from build123d import *

# Parameters (mm, degrees)
SKETCH1_R           = 15
BOSS_EXTRUDE1_DEPTH = 5
SKETCH3_R           = 18.5
SKETCH3_R_2         = 15
BOSS_EXTRUDE3_DEPTH = 1
SKETCH2_R           = 7.5
BOSS_EXTRUDE2_DEPTH = 0.5
BOSS_EXTRUDE5_DEPTH = 5.5
BOSS_EXTRUDE6_START = 0.5
BOSS_EXTRUDE6_DEPTH = 0.5


with BuildPart() as part:
    # Sketch1 → Boss-Extrude1 (new, symmetric)
    with BuildSketch(Plane.XY):
        with Locations((-2.17, 0)):
            Circle(SKETCH1_R)
        Polygon((-2, 3.464101615), (-4, 0), (-2, -3.464101615), (2, -3.464101615), (4, 0), (2, 3.464101615), align=None, mode=Mode.SUBTRACT)
    extrude(amount=BOSS_EXTRUDE1_DEPTH, both=True)

    # Sketch3 → Boss-Extrude3 (add)
    # profile 1 of 2: a face of its own
    with BuildSketch(Plane(origin=(0, 0, -5), x_dir=(-1, 0, 0), z_dir=(0, 0, -1))):
        with Locations((2.17, 0)):
            Circle(SKETCH3_R)
        with Locations(Location((2.17, 0, 0), (0, 0, 180))):
            Circle(SKETCH3_R_2, mode=Mode.SUBTRACT)
    # profile 2 of 2: a face of its own
    with BuildSketch(Plane(origin=(0, 0, -5), x_dir=(-1, 0, 0), z_dir=(0, 0, -1))):
        with Locations(Location((2.17, 0, 0), (0, 0, 180))):
            Circle(SKETCH3_R_2)
        Polygon((-4, 0), (-2, 3.464101615), (2, 3.464101615), (4, 0), (2, -3.464101615), (-2, -3.464101615), align=None, mode=Mode.SUBTRACT)
    extrude(amount=BOSS_EXTRUDE3_DEPTH)

    # Sketch2 → Boss-Extrude2 (add)
    with BuildSketch(Plane(origin=(0, 0, -6), x_dir=(-1, 0, 0), z_dir=(0, 0, -1))):
        Circle(SKETCH2_R)
        Polygon((2, -3.464101615), (-2, -3.464101615), (-4, 0), (-2, 3.464101615), (2, 3.464101615), (4, 0), align=None, mode=Mode.SUBTRACT)
    extrude(amount=BOSS_EXTRUDE2_DEPTH)

    # Sketch4 → Boss-Extrude5 (add)
    with BuildSketch(Plane.XY.offset(5)):
        Polygon((4, 6.92820323), (-4, 6.92820323), (-8, 0), (-4, -6.92820323), (4, -6.92820323), (8, 0), align=None)
    extrude(amount=BOSS_EXTRUDE5_DEPTH)

    # Sketch5 → Boss-Extrude6 (add)
    with BuildSketch(Plane.XY.offset(5).offset(BOSS_EXTRUDE6_START)):
        with BuildLine():
            ThreePointArc((-13.508064516, -9.820809184), (-7.396562926, -14.059980085), (0, -14.842206709))
            Line((0, -14.842206709), (0, -6.92820323))
            Line((0, -6.92820323), (-4, -6.92820323))
            Line((-4, -6.92820323), (-8, 0))
            Line((-8, 0), (-4, 6.92820323))
            Line((-4, 6.92820323), (0, 6.92820323))
            Line((0, 6.92820323), (0, 14.842206709))
            ThreePointArc((0, 14.842206709), (-7.396562926, 14.059980085), (-13.508064516, 9.820809184))
            ThreePointArc((-13.508064516, 9.820809184), (-16.33, 0), (-13.508064516, -9.820809184))
        make_face()
    extrude(amount=-BOSS_EXTRUDE6_DEPTH)


solid = part.part
Input: part model. Units: mm. Frame: model coordinates. A direction names the side the tool comes from. Coordinates: 2 decimals unless noted, no trailing zeros. Loops run counter-clockwise (first coordinate to the right, second up) from the corner with the lowest first, then second, coordinate; pieces in that order, holes last. Notation, with made-up numbers: (56, 35) -> (91, 35) arc R14 ccw to (91, 45) -> close; hole circle Ø9 at (-8.5, 8). An arc over 180 degrees is marked (long way). Write item = value, one per line. Start each with the question number.
Item 1: Reachability of faces 5 (the face through (-8.3, 0.2, 5.5)), 6 (the face through (-6.028, -3.416, 7.965)), 7 (the face through (-3.014, -1.708, -0.67)), 8 (the face through (6.028, 3.416, 7.712)), 9 (the face through (9, 0, 5)) from +Z, -Z, +X, -X, +Y, -Y: full face, straight path, thin tool, end or side. Return the list, or none.
Item 2: First-contact query: P1, Ø4.5, axis at x = 0.5, z = -0.5, coming from the +Y side; P2, Ø6, axis at x = 11.5, z = -0.5, coming from the +Y side; P3, Ø1.5, axis at x = 12, y = -1.5, coming from the +Z side. Flat tips, straight axial feed; report the tip coordinate or a pass-through.
Item 3: Cut plane B-B, the plane z = 6.5. Return loops of the section in (x, y).
Item 4: Mould query, pull axis Y, two halves, no side actions, for faces 1 (the face through (3.014, 1.708, -0.67)), 2 (the face through (-16.33, 0.14, 5.25)), 3 (the face through (-3.2, 1.8, -6.5)), 4 (the face through (-5.972, 3.513, 7.965)). Classes: pulls with the +Y half, pulls with the -Y half, needs draft (parallel to the pull), parting line crosses it, or undercut.
Item 5: Cut plane C-C, the plane y = -4.5. Return loops of the section in (x, z).
Item 6: Cut plane D-D, the plane x = -9. Return loops of the section in (y, z).
Item 7: Material intervals for line 1 (Z direction, x = 7, y = 14); line 2 (X direction, y = -1, z = 3); line 3 (Z direction, x = 11, y = 2.5), sorted ascending.
Item 8: Cut plane A-A, the plane z = -3. Return loops of the section in (x, y), plus the area to 3 significant figures.
Ans:
q1.face_5 = +Z, -X
q1.face_6 = +Z, -X, -Y
q1.face_7 = -Z
q1.face_8 = +Z, +X, +Y
q1.face_9 = +Z, +X
q2.P1 = 14.99
q2.P2 = 10.54
q2.P3 = 5
q3.outline = (-8, 0) -> (-4, -6.93) -> (4, -6.93) -> (8, 0) -> (4, 6.93) -> (-4, 6.93) -> close
q4.face_1 = undercut
q4.face_2 = parting line crosses it
q4.face_3 = needs draft
q4.face_4 = pulls with the +Y half
q5.outline = (-20.11, -6) -> (-6, -6) -> (-6, -6.5) -> (6, -6.5) -> (6, -6) -> (15.77, -6) -> (15.77, -5) -> (12.14, -5) -> (12.14, 5) -> (5.4, 5) -> (5.4, 10.5) -> (-5.4, 10.5) -> (-5.4, 5.5) -> (-15.77, 5.5) -> (-15.77, 5) -> (-16.48, 5) -> (-16.48, -5) -> (-20.11, -5) -> close
q6.outline = (-17.19, -6) -> (17.19, -6) -> (17.19, -5) -> (13.35, -5) -> (13.35, 5.5) -> (-13.35, 5.5) -> (-13.35, -5) -> (-17.19, -5) -> close
q7.line_1 = -6 to -5
q7.line_2 = -17.14 to -3.42, 3.42 to 12.8
q7.line_3 = -6 to 5
q8.outline = circle Ø30 at (-2.17, 0); hole (-4, 0) -> (-2, -3.46) -> (2, -3.46) -> (4, 0) -> (2, 3.46) -> (-2, 3.46) -> close
q8.area = 665 mm²
